Geometry check sheet. Reference: the model listing, model coordinates, mm. A direction names the side the tool comes from. Give positions to 0.01 mm unless a question says otherwise; leave off trailing zeros. Write each loop counter-clockwise with the first axis right and the second up, starting at its lowest first coordinate (ties: lowest second). Pieces come first, ordered by that corner, then holes. Notation, with made-up numbers: (16, 82.25) - (63, 82.25) arc R30 cw to (63, 120.25) - close; hole circle Ø11 at (6.25, 29). An arc over 180 degrees is marked (long way). One line per question, with ' | ' between items. Start each with the question number.
Q1. Set-up check for faces 1 (the face through (-25, 12.7, 0)), 2 (the face through (12.7, -26, 0)), 3 (the face through (12.7, 25, 0)), 4 (the face through (38.1, 0, 0)): record each of +Z, -Z, +X, -X, +Y, -Y from which the full face is reachable in a straight line by a thin tool's end or side.
Q2. Section check A-A on z = 1.75. Count the separate pieces of the cut face and the enclosed holes in it, and give its area (3 significant figures).
Q3. Section check B-B on x = 25.4. Record the boundary of the cut face in (y, z).
Q4. Section check C-C on y = 2.5. Record the boundary of the cut face in (x, z).
Q5. Gauge pin test, flat ends, axial feed: P1, Ø5, axis at y = -27, z = 1, coming from the +X side; P2, Ø2, axis at y = -15.5, z = -3, coming from the -X side; P3, Ø1.5, axis at x = 12.5, z = 2, coming from the -Y side. Record the tip position at first contact, or that the pin passes through.
Q6. Thickness scan on L1, parallel to Y at x = 0, z = 1.45; L2, parallel to X at y = 25.4, z = -2.15; L3, parallel to Y at x = 2, z = 2. Record the ranges inside material, lowest first. Write a range as [from, to].
Q7. Section check D-D on x = 1. Record the boundary of the cut face in (y, z).
```python
from build123d import *

# Parameters (mm, degrees)
F0_R     = 12.7
F0_R_2   = 11.049
F1_DEPTH = 4.7625
F2_R     = 11.049
F3_DEPTH = 4.7625
F4_R     = 5.08


with BuildPart() as f1:
    # F0 (on Top) → F1 (new body, symmetric)
    with BuildSketch(Plane.XY):
        Circle(F0_R)
        Circle(F0_R_2, mode=Mode.SUBTRACT)
    extrude(amount=F1_DEPTH, both=True)

    # F2 (on Top) → F3 (join, symmetric)
    with BuildSketch(Plane.XY):
        with BuildLine():
            Line((0, 38.1), (-12.7, 38.1))
            Line((-12.7, 38.1), (-12.7, 25.4))
            ThreePointArc((-12.7, 25.4), (-8.980256, 34.380256), (0, 38.1))
        make_face()
        with BuildLine():
            Line((12.7, 38.1), (0, 38.1))
            ThreePointArc((0, 38.1), (8.980256, 34.380256), (12.7, 25.4))
            Line((12.7, 25.4), (12.7, 38.1))
        make_face()
        with BuildLine():
            ThreePointArc((11.049, 25.4), (-7.812823, 33.212823), (0, 14.351))
            ThreePointArc((0, 14.351), (7.812823, 17.587177), (11.049, 25.4))
        make_face()
        with BuildLine():
            ThreePointArc((12.7, 25.4), (8.980256, 34.380256), (0, 38.1))
            ThreePointArc((0, 38.1), (-8.980256, 34.380256), (-12.7, 25.4))
            ThreePointArc((-12.7, 25.4), (-8.980256, 16.419744), (0, 12.7))
            ThreePointArc((0, 12.7), (8.980256, 16.419744), (12.7, 25.4))
        make_face()
        with BuildLine():
            ThreePointArc((11.049, 25.4), (7.812823, 17.587177), (0, 14.351))
            ThreePointArc((0, 14.351), (-7.812823, 33.212823), (11.049, 25.4))
        make_face(mode=Mode.SUBTRACT)
        with BuildLine():
            ThreePointArc((0, 12.7), (-8.980256, 16.419744), (-12.7, 25.4))
            Line((-12.7, 25.4), (-12.7, 12.7))
            Line((-12.7, 12.7), (-25.4, 12.7))
            ThreePointArc((-25.4, 12.7), (-16.419744, 8.980256), (-12.7, 0))
            ThreePointArc((-12.7, 0), (-8.980256, 8.980256), (0, 12.7))
        make_face()
        with BuildLine():
            Line((12.7, 12.7), (12.7, 25.4))
            ThreePointArc((12.7, 25.4), (8.980256, 16.419744), (0, 12.7))
            ThreePointArc((0, 12.7), (8.980256, 8.980256), (12.7, 0))
            ThreePointArc((12.7, 0), (16.419744, 8.980256), (25.4, 12.7))
            Line((25.4, 12.7), (12.7, 12.7))
        make_face()
        with Locations((-25.4, 0)):
            Circle(F2_R)
        with BuildLine():
            ThreePointArc((-12.7, 0), (-16.419744, 8.980256), (-25.4, 12.7))
            ThreePointArc((-25.4, 12.7), (-34.380256, 8.980256), (-38.1, 0))
            ThreePointArc((-38.1, 0), (-34.380256, -8.980256), (-25.4, -12.7))
            ThreePointArc((-25.4, -12.7), (-16.419744, -8.980256), (-12.7, 0))
        make_face()
        with Locations((-25.4, 0)):
            Circle(F2_R, mode=Mode.SUBTRACT)
        with BuildLine():
            ThreePointArc((-38.1, 0), (-34.380256, 8.980256), (-25.4, 12.7))
            Line((-25.4, 12.7), (-38.1, 12.7))
            Line((-38.1, 12.7), (-38.1, 0))
        make_face()
        with BuildLine():
            ThreePointArc((36.449, 0), (25.4, 11.049), (14.351, 0))
            ThreePointArc((14.351, 0), (25.4, -11.049), (36.449, 0))
        make_face()
        with BuildLine():
            ThreePointArc((25.4, 12.7), (16.419744, 8.980256), (12.7, 0))
            ThreePointArc((12.7, 0), (16.419744, -8.980256), (25.4, -12.7))
            ThreePointArc((25.4, -12.7), (34.380256, -8.980256), (38.1, 0))
            ThreePointArc((38.1, 0), (34.380256, 8.980256), (25.4, 12.7))
        make_face()
        with BuildLine():
            ThreePointArc((36.449, 0), (25.4, -11.049), (14.351, 0))
            ThreePointArc((14.351, 0), (25.4, 11.049), (36.449, 0))
        make_face(mode=Mode.SUBTRACT)
        with BuildLine():
            ThreePointArc((25.4, -12.7), (16.419744, -8.980256), (12.7, 0))
            ThreePointArc((12.7, 0), (8.980256, -8.980256), (0, -12.7))
            ThreePointArc((0, -12.7), (8.980256, -16.419744), (12.7, -25.4))
            Line((12.7, -25.4), (12.7, -12.7))
            Line((12.7, -12.7), (25.4, -12.7))
        make_face()
        with BuildLine():
            ThreePointArc((0, -12.7), (-8.980256, -8.980256), (-12.7, 0))
            ThreePointArc((-12.7, 0), (-16.419744, -8.980256), (-25.4, -12.7))
            Line((-25.4, -12.7), (-12.7, -12.7))
            Line((-12.7, -12.7), (-12.7, -25.4))
            ThreePointArc((-12.7, -25.4), (-8.980256, -16.419744), (0, -12.7))
        make_face()
        with BuildLine():
            Line((38.1, 12.7), (25.4, 12.7))
            ThreePointArc((25.4, 12.7), (34.380256, 8.980256), (38.1, 0))
            Line((38.1, 0), (38.1, 12.7))
        make_face()
        with BuildLine():
            ThreePointArc((-25.4, -12.7), (-34.380256, -8.980256), (-38.1, 0))
            Line((-38.1, 0), (-38.1, -12.7))
            Line((-38.1, -12.7), (-25.4, -12.7))
        make_face()
        with BuildLine():
            ThreePointArc((38.1, 0), (34.380256, -8.980256), (25.4, -12.7))
            Line((25.4, -12.7), (38.1, -12.7))
            Line((38.1, -12.7), (38.1, 0))
        make_face()
        with BuildLine():
            ThreePointArc((11.049, -25.4), (7.812823, -17.587177), (0, -14.351))
            ThreePointArc((0, -14.351), (-7.812823, -33.212823), (11.049, -25.4))
        make_face()
        with BuildLine():
            ThreePointArc((12.7, -25.4), (8.980256, -16.419744), (0, -12.7))
            ThreePointArc((0, -12.7), (-8.980256, -16.419744), (-12.7, -25.4))
            ThreePointArc((-12.7, -25.4), (-8.980256, -34.380256), (0, -38.1))
            ThreePointArc((0, -38.1), (8.980256, -34.380256), (12.7, -25.4))
        make_face()
        with BuildLine():
            ThreePointArc((11.049, -25.4), (-7.812823, -33.212823), (0, -14.351))
            ThreePointArc((0, -14.351), (7.812823, -17.587177), (11.049, -25.4))
        make_face(mode=Mode.SUBTRACT)
        with BuildLine():
            Line((12.7, -38.1), (12.7, -25.4))
            ThreePointArc((12.7, -25.4), (8.980256, -34.380256), (0, -38.1))
            Line((0, -38.1), (12.7, -38.1))
        make_face()
        with BuildLine():
            ThreePointArc((0, -38.1), (-8.980256, -34.380256), (-12.7, -25.4))
            Line((-12.7, -25.4), (-12.7, -38.1))
            Line((-12.7, -38.1), (0, -38.1))
        make_face()
    extrude(amount=F3_DEPTH, both=True)

    # F4
    f4_edges = [f1.edges().sort_by_distance(p)[0] for p in [
        (12.7, -12.7, 0),
        (12.7, -38.1, 0),
        (-12.7, -38.1, 0),
        (38.1, -12.7, 0),
        (38.1, 12.7, 0),
        (12.7, 38.1, 0),
        (-38.1, 12.7, 0),
        (-12.7, 38.1, 0),
        (12.7, 12.7, 0),
        (-12.7, 12.7, 0),
        (-38.1, -12.7, 0),
        (-12.7, -12.7, 0),
    ]]
    fillet(f4_edges, radius=F4_R)


solid = f1.part
```
Working result:
1) face 1: +Z, -Z, -X, +Y | face 2: +Z, -Z, +X, -Y | face 3: +Z, -Z, +X, +Y | face 4: +Z, -Z, +X, +Y, -Y
2) separate pieces: 1 | enclosed holes: 5 | area: 1,290 mm2
3) outline: (-12.7, -4.76) - (-11.05, -4.76) - (-11.05, 4.76) - (-12.7, 4.76) - close; (11.05, -4.76) - (12.7, -4.76) - (12.7, 4.76) - (11.05, 4.76) - close
4) outline: (-38.1, -4.76) - (-36.16, -4.76) - (-36.16, 4.76) - (-38.1, 4.76) - close; (-14.64, -4.76) - (-10.76, -4.76) - (-10.76, 4.76) - (-14.64, 4.76) - close; (10.76, -4.76) - (14.64, -4.76) - (14.64, 4.76) - (10.76, 4.76) - close; (36.16, -4.76) - (38.1, -4.76) - (38.1, 4.76) - (36.16, 4.76) - close
5) P1: stops at x = 12.7 | P2: stops at x = -13.9 | P3: stops at y = -35.98
6) L1: y = [-38.1, -36.45], [-14.35, -11.05], [11.05, 14.35], [36.45, 38.1] | L2: x = [-12.7, -11.05], [11.05, 12.7] | L3: y = [-38.1, -36.27], [-14.53, -10.87], [10.87, 14.53], [36.27, 38.1]
7) outline: (-38.1, -4.76) - (-36.4, -4.76) - (-36.4, 4.76) - (-38.1, 4.76) - close; (-14.4, -4.76) - (-11, -4.76) - (-11, 4.76) - (-14.4, 4.76) - close; (11, -4.76) - (14.4, -4.76) - (14.4, 4.76) - (11, 4.76) - close; (36.4, -4.76) - (38.1, -4.76) - (38.1, 4.76) - (36.4, 4.76) - close
